```python
from build123d import *

# Parameters (mm, degrees)
SKETCH4_W           = 13.5
SKETCH4_H           = 15.3
SKETCH4_W_2         = 12
SKETCH4_H_2         = 13.8
BOSS_EXTRUDE1_DEPTH = 2.7
SKETCH5_W           = 13.5
SKETCH5_H           = 15.3
BOSS_EXTRUDE2_DEPTH = 1
SKETCH6_W           = 24
SKETCH6_H           = 0.75
BOSS_EXTRUDE3_DEPTH = 4
CUT_EXTRUDE1_REACH  = 22.566
SKETCH8_W           = 5.25
SKETCH8_H           = 0.75
BOSS_EXTRUDE4_DEPTH = 3.7
SKETCH9_W           = 5.25
SKETCH9_H           = 0.75
BOSS_EXTRUDE5_DEPTH = 3.7
SKETCH10_W          = 13.5
SKETCH10_H          = 3.7
BOSS_EXTRUDE6_DEPTH = 2
CHAMFER1_SIZE       = 2.7
CHAMFER1_SIZE_2     = 0.9
SKETCH11_W          = 16.55
SKETCH11_H          = 3.7
BOSS_EXTRUDE7_DEPTH = 1
SKETCH12_W          = 16.55
SKETCH12_H          = 3.7
BOSS_EXTRUDE8_DEPTH = 1
CUT_EXTRUDE2_REACH  = 24.114


with BuildPart() as part:
    # Sketch4 → Boss-Extrude1 (new body)
    with BuildSketch(Plane(origin=(0, 0, 0), x_dir=(1, 0, 0), z_dir=(0, 1, 0))):
        with Locations((0, -7.674098898)):
            Rectangle(SKETCH4_W, SKETCH4_H)
        with Locations((0, -7.674098898)):
            Rectangle(SKETCH4_W_2, SKETCH4_H_2, mode=Mode.SUBTRACT)
    extrude(amount=BOSS_EXTRUDE1_DEPTH)

    # Sketch5 → Boss-Extrude2 (add)
    with BuildSketch(Plane.XZ):
        with Locations((0, 7.674098898)):
            Rectangle(SKETCH5_W, SKETCH5_H)
    extrude(amount=BOSS_EXTRUDE2_DEPTH)

    # Sketch6 → Boss-Extrude3 (add)
    with BuildSketch(Plane(origin=(0, 2.7, 0), x_dir=(1, 0, 0), z_dir=(0, 1, 0))):
        with Locations((0, -0.399098898)):
            Rectangle(SKETCH6_W, SKETCH6_H)
    extrude(amount=BOSS_EXTRUDE3_DEPTH)

    # Sketch7 → Cut-Extrude1 (cut, up to next)
    with BuildSketch(Plane(origin=(0, 0, 0.024098898), x_dir=(-1, 0, 0), z_dir=(0, 0, -1)), mode=Mode.PRIVATE) as cut_extrude1_sk1:
        with BuildLine():
            Line((-4.5, 0.919), (4.5, 0.919))
            ThreePointArc((4.5, 0.919), (4.853553391, 1.065446609), (5, 1.419))
            Line((5, 1.419), (5, 3.919))
            ThreePointArc((5, 3.919), (4.853553391, 4.272553391), (4.5, 4.419))
            Line((4.5, 4.419), (-4.5, 4.419))
            ThreePointArc((-4.5, 4.419), (-4.853553391, 4.272553391), (-5, 3.919))
            Line((-5, 3.919), (-5, 1.419))
            ThreePointArc((-5, 1.419), (-4.853553391, 1.065446609), (-4.5, 0.919))
        make_face()
    cut_extrude1_tool1 = extrude(cut_extrude1_sk1.sketch, amount=-CUT_EXTRUDE1_REACH, mode=Mode.PRIVATE) & part.part
    add(cut_extrude1_tool1.solids().sort_by_distance((0, 2.669, 0.024099))[0], mode=Mode.SUBTRACT)

    # Sketch8 → Boss-Extrude4 (add)
    with BuildSketch(Plane.XZ.offset(-2.7)):
        with Locations((9.375, 0.399098898)):
            Rectangle(SKETCH8_W, SKETCH8_H)
    extrude(amount=BOSS_EXTRUDE4_DEPTH)

    # Sketch9 → Boss-Extrude5 (add)
    with BuildSketch(Plane.XZ.offset(-2.7)):
        with Locations((-9.375, 0.399098898)):
            Rectangle(SKETCH9_W, SKETCH9_H)
    extrude(amount=BOSS_EXTRUDE5_DEPTH)

    # Sketch10 → Boss-Extrude6 (add)
    with BuildSketch(Plane.XY.offset(15.324098898)):
        with Locations((0, 0.85)):
            Rectangle(SKETCH10_W, SKETCH10_H)
    extrude(amount=BOSS_EXTRUDE6_DEPTH)

    # Chamfer1
    # the kernel refuses this chamfer: 2.7, 0.9 mm, written as the material it takes off along each edge
    with BuildSketch(Plane(origin=(-6, 2.7, 14.574098898), x_dir=(0, -0.9999257509361695, -0.012185754582199112), z_dir=(1, 0, 0))) as chamfer1_piece_1:
        Polygon((CHAMFER1_SIZE * 0.999925750936, -CHAMFER1_SIZE * 0.0121857545822), (-CHAMFER1_SIZE_2 * 0.0121857545822, -CHAMFER1_SIZE_2 * 0.999925750936), (0, 0), align=None)
    extrude(amount=12, mode=Mode.SUBTRACT)

    # Sketch11 → Boss-Extrude7 (add)
    with BuildSketch(Plane(origin=(6.75, 0, 0), x_dir=(0, 0, -1), z_dir=(1, 0, 0))):
        with Locations((-9.049098898, 0.85)):
            Rectangle(SKETCH11_W, SKETCH11_H)
    extrude(amount=BOSS_EXTRUDE7_DEPTH)

    # Sketch12 → Boss-Extrude8 (add)
    with BuildSketch(Plane.ZY.offset(6.75)):
        with Locations((9.049098898, 0.85)):
            Rectangle(SKETCH12_W, SKETCH12_H)
    extrude(amount=BOSS_EXTRUDE8_DEPTH)

    # Sketch13 → Cut-Extrude2 (cut, up to next)
    with BuildSketch(Plane(origin=(0, 0, 0), x_dir=(1, 0, 0), z_dir=(0, 1, 0)), mode=Mode.PRIVATE) as cut_extrude2_sk1:
        with BuildLine():
            Line((-4.5, -12.174098898), (4.5, -12.174098898))
            ThreePointArc((4.5, -12.174098898), (4.853553391, -12.320545507), (5, -12.674098898))
            Line((5, -12.674098898), (5, -13.074098898))
            ThreePointArc((5, -13.074098898), (4.853553391, -13.427652289), (4.5, -13.574098898))
            Line((4.5, -13.574098898), (-4.5, -13.574098898))
            ThreePointArc((-4.5, -13.574098898), (-4.853553391, -13.427652289), (-5, -13.074098898))
            Line((-5, -13.074098898), (-5, -12.674098898))
            ThreePointArc((-5, -12.674098898), (-4.853553391, -12.320545507), (-4.5, -12.174098898))
        make_face()
    cut_extrude2_tool1 = extrude(cut_extrude2_sk1.sketch, amount=-CUT_EXTRUDE2_REACH, mode=Mode.PRIVATE) & part.part
    add(cut_extrude2_tool1.solids().sort_by_distance((0, 0, 12.874099))[0], mode=Mode.SUBTRACT)


solid = part.part
```
Source: CAD feature listing. Evaluate the final solid. Frame: model axes, mm. A direction names the side the tool comes from. Give positions to 0.01 mm unless a question says otherwise; leave off trailing zeros. Loops run counter-clockwise (first coordinate to the right, second up) from the corner with the lowest first, then second, coordinate; pieces in that order, holes last. Notation, with made-up numbers: (35, -37) -> (42, -37) arc R8 ccw to (42, -24) -> close; hole circle Ø3 at (83, 72). An arc over 180 degrees is marked (long way). Use a Markdown table: item, result. Add a question column.
(1) Ray query, line 1 (X direction, y = 1.75, z = 2); line 2 (Y direction, x = 2.25, z = 8); line 3 (Y direction, x = 3.25, z = 16). Return the intervals inside material, ascending.
(2) Section query C-C (y = 3.25). Output: boundary loops of the cut face in (x, z).
(3) Pull-direction query (X, two-part tool) for faces 5 (the face through (0, 0, 8)), 6 (the face through (0, 5, 0.024)), 7 (the face through (0.1, -0.5, 13.574)), 8 (the face through (7.75, 1, 9)); classes: +X half, -X half, draft (parallel to the pull), parting line (faces both ways), or undercut.
(4) Section query D-D (z = 7.25). Output: boundary loops of the cut face in (x, y), then the cut area to 4 significant figures.
(5) First-contact query: pin 1 Ø4 at (y, z) = (1.5, 6) entering from +X; pin 2 Ø4.5 at (x, z) = (-2, 10) entering from +Y; pin 3 Ø1.5 at (y, z) = (5.5, 3.5) entering from -X; pin 4 Ø1.4 at (y, z) = (1.5, 6) entering from -X. Flat tips, straight axial feed; report the tip coordinate or a pass-through.
(6) Access query for faces 1 (the face through (-7.75, 1, 9)), 2 (the face through (-1, 2.7, 16)), 3 (the face through (-0.1, -0.5, 12.174)), 4 (the face through (-6, 1, 8)). Directions: +Z, -Z, +X, -X, +Y, -Y. A direction counts if a zero-diameter tool reaches every point of the face in a straight line with its end or side. Return the directions, or none.
(7) Section query B-B (x = 2.25). Output: boundary loops of the cut face in (y, z).
Checked values:
| question | item | result |
|---|---|---|
| 1 | line 1 | -7.75 to -6, 6 to 7.75 |
| 1 | line 2 | -1 to 0 |
| 1 | line 3 | -1 to 2.7 |
| 2 | outline | (-12, 0.02) -> (-5, 0.02) -> (-5, 0.77) -> (-12, 0.77) -> close; (5, 0.02) -> (12, 0.02) -> (12, 0.77) -> (5, 0.77) -> close |
| 3 | face 5 | undercut |
| 3 | face 6 | draft |
| 3 | face 7 | undercut |
| 3 | face 8 | +X half |
| 4 | outline | (-7.75, -1) -> (7.75, -1) -> (7.75, 2.7) -> (6, 2.7) -> (6, 0) -> (-6, 0) -> (-6, 2.7) -> (-7.75, 2.7) -> close |
| 4 | area | 24.95 mm^2 |
| 5 | pin 1 | x = 7.75 |
| 5 | pin 2 | y = 0 |
| 5 | pin 3 | through |
| 5 | pin 4 | x = -7.75 |
| 6 | face 1 | +Z, -X, +Y, -Y |
| 6 | face 2 | +Z, +X, -X, +Y |
| 6 | face 3 | +Y, -Y |
| 6 | face 4 | +Y |
| 7 | outline | (-1, 0.02) -> (0.92, 0.02) -> (0.92, 0.77) -> (0, 0.77) -> (0, 12.17) -> (-1, 12.17) -> close; (-1, 13.57) -> (0, 13.57) -> (0, 14.57) -> (2.7, 15.47) -> (2.7, 17.32) -> (-1, 17.32) -> close; (4.42, 0.02) -> (6.7, 0.02) -> (6.7, 0.77) -> (4.42, 0.77) -> close |
